```python
from build123d import *

# Parameters (mm, degrees)
F1_DEPTH = 100
F2_R     = 20
F3_R     = 10
F4_SIZE  = 10
F5_SIZE  = 2


with BuildPart() as f1:
    # F0 (on Top) → F1 (new body)
    with BuildSketch(Plane.XY):
        Polygon((-15, 0), (0, 0), (0, 200), (-15, 200), (-15, 130), (-60, 130), (-60, 112.5), (-188, 112.5), (-188, 87.5), (-60, 87.5), (-60, 70), (-15, 70), align=None)
    extrude(amount=F1_DEPTH)

    # F2
    f2_edges = [f1.edges().sort_by_distance(p)[0] for p in [
        (-15, 70, 50),
        (-15, 130, 50),
    ]]
    fillet(f2_edges, radius=F2_R)

    # F3
    f3_edges = [f1.edges().sort_by_distance(p)[0] for p in [
        (-60, 87.5, 50),
        (-60, 112.5, 50),
    ]]
    fillet(f3_edges, radius=F3_R)

    # F4
    f4_edges = [f1.edges().sort_by_distance(p)[0] for p in [
        (-7.5, 200, 100),
        (-7.5, 0, 100),
        (-7.5, 0, 0),
        (-7.5, 200, 0),
    ]]
    chamfer(f4_edges, length=F4_SIZE)

    # F5
    f5_edges = [f1.edges().sort_by_distance(p)[0] for p in [
        (-60, 70, 50),
        (-60, 130, 50),
    ]]
    chamfer(f5_edges, length=F5_SIZE)


solid = f1.part
```
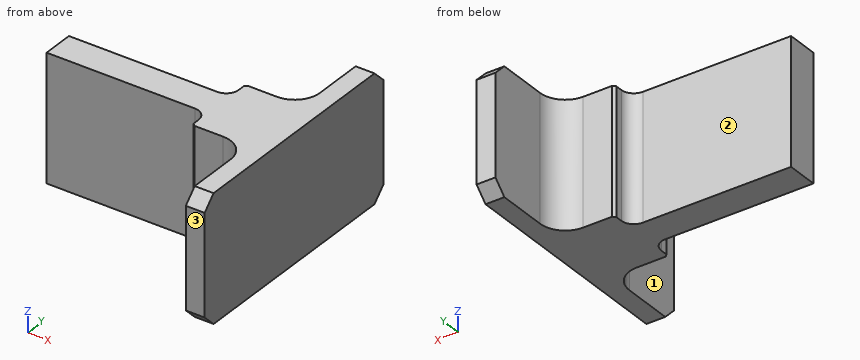
Could you check a few things on this model? Use its own coordinates, in mm. Face numbers are marked on the shaded views. A direction names the side the tool comes from. Give positions to 0.01 mm unless a question says otherwise; leave off trailing zeros. Loops run counter-clockwise (first coordinate to the right, second up) from the corner with the lowest first, then second, coordinate; pieces in that order, holes last. Notation, with made-up numbers: (84, 16) - (137, 16) arc R18 cw to (137, 48) - close; hole circle Ø6 at (-0.75, 44.25). An arc over 180 degrees is marked (long way). Answer in a Markdown table with one row per item. Add a question column.
Q1. Please list where these lines run through material, in increasing order: L1, parallel to Y at x = -47.5, z = 15.5; L2, parallel to X at y = 75, z = 15; L3, parallel to X at y = 32, z = 66. Write a range as from..to.
Q2. For pin 1 (1.5 mm diameter, centred on y = 172, z = 27, fed in from -X); pin 2 (2 mm diameter, centred on x = -151, z = 35, fed in from -Y); pin 3 (2 mm diameter, centred on x = -95, z = 42.5, fed in from +Y), each with a flat end and sliding along its axis, tell me the tip position at first contact or that it passes through.
Q3. Which directions (+Z, -Z, +X, -X, +Y, -Y) give clear straight access to the entire face, cutting with the end or side of a thin tool? Please do the marked faces 1, 2 and 3.
Q4. If we section it at A-A (z = 75): List the corners of the cut face in (x, y) for me.
Q5. If we section it at C-C (x = -105): List the corners of the cut face in (y, z) for me, plus the area to 3 significant figures.
Q6. If we section it at B-B (y = 29.5): List the corners of the cut face in (x, z) for me.
The answers:
| question | item | result |
|---|---|---|
| 1 | L1 | y = 70..130 |
| 1 | L2 | x = -60..0 |
| 1 | L3 | x = -15..0 |
| 2 | pin 1 | stops at x = -15 |
| 2 | pin 2 | stops at y = 87.5 |
| 2 | pin 3 | stops at y = 112.5 |
| 3 | face 1 | +Z, -Z, -X, -Y |
| 3 | face 2 | +Z, -Z, -X, +Y |
| 3 | face 3 | +Z, -Z, +X, -X, -Y |
| 4 | outline | (-188, 87.5) - (-70, 87.5) arc R10 cw to (-60, 77.5) - (-60, 72) - (-58, 70) - (-35, 70) arc R20 cw to (-15, 50) - (-15, 0) - (0, 0) - (0, 200) - (-15, 200) - (-15, 150) arc R20 cw to (-35, 130) - (-58, 130) - (-60, 128) - (-60, 122.5) arc R10 cw to (-70, 112.5) - (-188, 112.5) - close |
| 5 | outline | (87.5, 0) - (112.5, 0) - (112.5, 100) - (87.5, 100) - close |
| 5 | area | 2,500 mm^2 |
| 6 | outline | (-15, 0) - (0, 0) - (0, 100) - (-15, 100) - close |
